Design review of the part shown in the three views and the two pictorial views. Dimensions are in mm from the part's minimum x, y and z. A direction names the side the tool comes from. Round coordinates to 2 decimals unless told otherwise and drop trailing zeros. Write each loop counter-clockwise with the first axis right and the second up, starting at its lowest first coordinate (ties: lowest second). Pieces come first, ordered by that corner, then holes. Notation, with made-up numbers: (25, 39.5) - (77, 39.5) arc R18 ccw to (77, 60.5) - close; hole circle Ø4 at (31.25, -16.75). An arc over 180 degrees is marked (long way). Use one line per item in the form item = value.
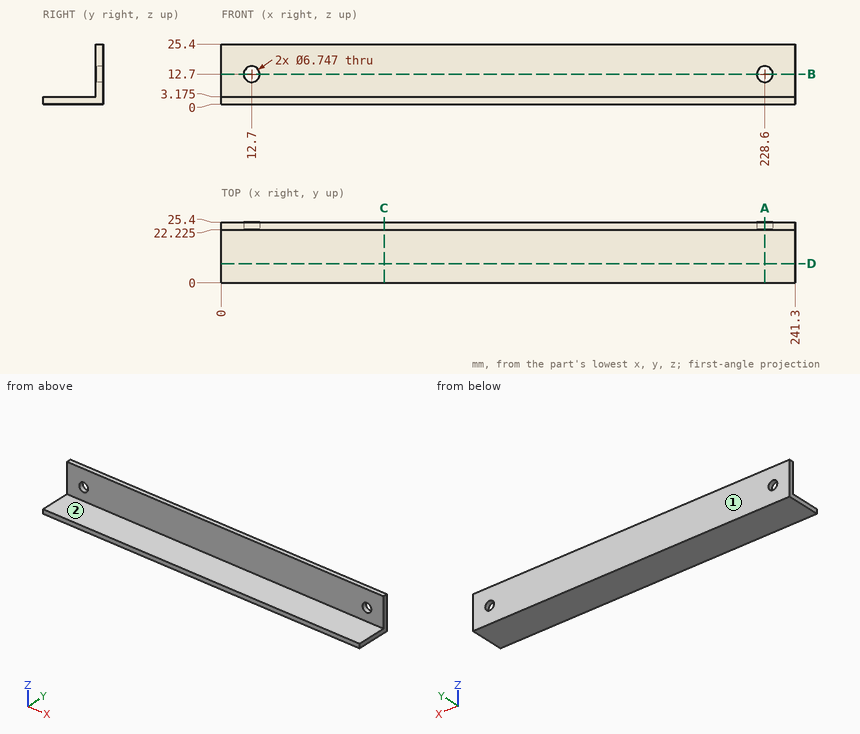
Q1. We need section A-A on x = 228.6. Write out the cut boundary in (y, z) (1 decimal), then the cut area to 3 significant figures.
Calculated:
outline = (0, 0) - (25.4, 0) - (25.4, 9.3) - (22.2, 9.3) - (22.2, 3.2) - (0, 3.2) - close; (22.2, 16.1) - (25.4, 16.1) - (25.4, 25.4) - (22.2, 25.4) - close
area = 130 mm2
Q2. For P1, Ø5.5, axis at x = 12.7, z = 12.7, coming from the +Y side; P2, Ø1, axis at x = 120, y = 19, coming from the +Z side (3 decimals); P3, Ø10, axis at x = 194.5, z = 20, coming from the -Y side (3 decimals); P4, Ø3, axis at x = 36.5, y = 16, coming from the -Z side, all flat-tipped, find the tip position at first contact; note any pin that passes through.
Calculated:
P1 = through
P2 = 3.175
P3 = 22.225
P4 = 0
Q3. We need section C-C on x = 68.5. Write out the cut boundary in (y, z) (3 decimals), then the cut area to 3 significant figures.
Calculated:
outline = (0, 0) - (25.4, 0) - (25.4, 25.4) - (22.225, 25.4) - (22.225, 3.175) - (0, 3.175) - close
area = 151 mm2
Q4. To check wall thickness, follow line 1 along X through (y, z) = (24, 12.7); line 2 along Z through (x, y) = (12.7, 24.65); line 3 along Y through (x, z) = (148.5, 22.75) (3 decimals). State the ranges of each line that lie inside material, in increasing order. Write a range as from..to.
Calculated:
line_1 = 0..9.33, 16.07..225.23, 231.97..241.3
line_2 = 0..9.33, 16.07..25.4
line_3 = 22.225..25.4
Q5. We need section B-B on z = 12.7. Write out the cut boundary in (x, y) (1 decimal).
Calculated:
outline = (0, 22.2) - (9.3, 22.2) - (9.3, 25.4) - (0, 25.4) - close; (16.1, 22.2) - (225.2, 22.2) - (225.2, 25.4) - (16.1, 25.4) - close; (232, 22.2) - (241.3, 22.2) - (241.3, 25.4) - (232, 25.4) - close
Q6. We need section D-D on y = 8. Write out the cut boundary in (x, z) (3 decimals), then the cut area to 3 significant figures.
Calculated:
outline = (0, 0) - (241.3, 0) - (241.3, 3.175) - (0, 3.175) - close
area = 766 mm2
Q7. Machinability: for the marked faces 1 and 2, which of the approach directions +Z, -Z, +X, -X, +Y, -Y give a long, thin tool a straight path to every point of the face, cutting with its end or side? Answer none if there is none.
Calculated:
face_1 = +Z, -Z, +X, -X, +Y
face_2 = +Z, +X, -X, -Y
